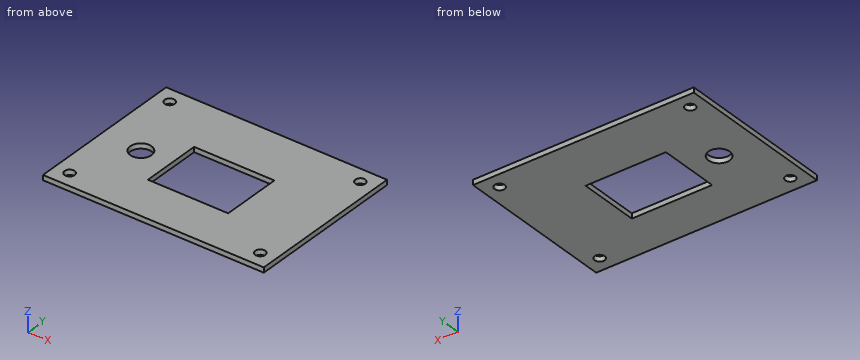
```python
from build123d import *

# Parameters (mm, degrees)
F0_W     = 139.7
F0_H     = 101.6
F0_R     = 3.175
F0_R_2   = 6.746875
F0_W_2   = 50.8
F0_H_2   = 38.1
F1_DEPTH = 3.175


# Not quite as in the source:
# - a feature names something its author has since deleted; it is built from what else it names


with BuildPart() as f1:
    # F0 (on Top) → F1 (new body)
    with BuildSketch(Plane.XY):
        with Locations((69.85, 50.8)):
            Rectangle(F0_W, F0_H)
        with Locations((9.525, 9.525)):
            Circle(F0_R, mode=Mode.SUBTRACT)
        with Locations((25.4, 47.625)):
            Circle(F0_R_2, mode=Mode.SUBTRACT)
        with Locations((130.175, 9.525)):
            Circle(F0_R, mode=Mode.SUBTRACT)
        with Locations((69.85, 47.625)):
            Rectangle(F0_W_2, F0_H_2, mode=Mode.SUBTRACT)
        with Locations((9.525, 92.075)):
            Circle(F0_R, mode=Mode.SUBTRACT)
        with Locations((130.175, 92.075)):
            Circle(F0_R, mode=Mode.SUBTRACT)
    extrude(amount=F1_DEPTH)


solid = f1.part
```
Geometry: final body of the model. Coordinates: model frame, mm. Round coordinates to 2 decimals unless told otherwise and drop trailing zeros. Loops run counter-clockwise (first coordinate to the right, second up) from the corner with the lowest first, then second, coordinate; pieces in that order, holes last. Notation, with made-up numbers: (66.5, -38.5) -> (109.5, -38.5) arc R21 ccw to (109.5, -31.5) -> close; hole circle Ø9 at (0.5, 50). An arc over 180 degrees is marked (long way). Use one line per item in the form item = value. Start each with the question number.
1) Section C-C on z = 2.05. Output: boundary loops of the cut face in (x, y) (3 decimals).
2) Line query: L1, parallel to X at y = 64, z = 2.55; L2, parallel to X at y = 46, z = 1.7; L3, parallel to Y at x = 57.5, z = 1.9 (3 decimals). Output: solid intervals per line, ascending.
3) Section A-A on x = 25.4. Output: boundary loops of the cut face in (y, z) (3 decimals), then the cut area to 3 significant figures.
4) First-contact query: P1, Ø1.5, axis at x = 19, y = 43, coming from the -Z side. Flat tip, straight axial feed; report the tip coordinate or a pass-through.
5) Section D-D on x = 69.5. Output: boundary loops of the cut face in (y, z) (3 decimals), then the cut area to 3 significant figures.
6) Section B-B on y = 45. Output: boundary loops of the cut face in (x, z) (3 decimals).
Response:
q1.outline = (0, 0) -> (139.7, 0) -> (139.7, 101.6) -> (0, 101.6) -> close; hole circle Ø6.35 at (9.525, 9.525); hole circle Ø6.35 at (9.525, 92.075); hole circle Ø13.494 at (25.4, 47.625); hole (44.45, 28.575) -> (95.25, 28.575) -> (95.25, 66.675) -> (44.45, 66.675) -> close; hole circle Ø6.35 at (130.175, 9.525); hole circle Ø6.35 at (130.175, 92.075)
q2.L1 = 0 to 44.45, 95.25 to 139.7
q2.L2 = 0 to 18.85, 31.95 to 44.45, 95.25 to 139.7
q2.L3 = 0 to 28.575, 66.675 to 101.6
q3.outline = (0, 0) -> (40.878, 0) -> (40.878, 3.175) -> (0, 3.175) -> close; (54.372, 0) -> (101.6, 0) -> (101.6, 3.175) -> (54.372, 3.175) -> close
q3.area = 280 mm^2
q4.P1 = 0
q5.outline = (0, 0) -> (28.575, 0) -> (28.575, 3.175) -> (0, 3.175) -> close; (66.675, 0) -> (101.6, 0) -> (101.6, 3.175) -> (66.675, 3.175) -> close
q5.area = 202 mm^2
q6.outline = (0, 0) -> (19.185, 0) -> (19.185, 3.175) -> (0, 3.175) -> close; (31.615, 0) -> (44.45, 0) -> (44.45, 3.175) -> (31.615, 3.175) -> close; (95.25, 0) -> (139.7, 0) -> (139.7, 3.175) -> (95.25, 3.175) -> close
